Check sheet for the modelled part. Datum: model origin and axes. Units: mm. A direction names the side the tool comes from. Give positions to 0.01 mm unless a question says otherwise; leave off trailing zeros. Loops run counter-clockwise (first coordinate to the right, second up) from the corner with the lowest first, then second, coordinate; pieces in that order, holes last. Notation, with made-up numbers: (13, -13.75) - (60, -13.75) arc R29 cw to (60, 24.25) - close; hole circle Ø7 at (-26, -9). An arc over 180 degrees is marked (long way). Answer in a Markdown table with one row per item. Add a question column.
(1) Sectioned sample at D-D on z = 20.5. Enter the section's corners in (x, y).
(2) Sectioned sample at C-C on y = 13. Enter the section's corners in (x, z), then the cut area to 3 significant figures.
(3) Go/stop test with flat-tipped pins: P1, Ø2, axis at y = 8, z = 2.5, coming from the +X side; P2, Ø2, axis at y = -5.5, z = 3.5, coming from the -X side; P3, Ø1, axis at x = -4, y = -6, coming from the +Z side; P4, Ø1.5, axis at x = -2, y = -3.5, coming from the -Z side. Record where each tip stops, or that it passes through.
(4) Sectioned sample at A-A on z = 6. Enter the section's corners in (x, y), then the cut area to 3 significant figures.
(5) Sectioned sample at B-B on y = -3.25. Enter the section's corners in (x, z), then the cut area to 3 significant figures.
(6) Set-up check for faces 4 (the face through (-6, 1, 11)), 5 (the face through (3.624, -1.945, 0.493)), 6 (the face through (-0.617, -5.4, 0.5)): record each of +Z, -Z, +X, -X, +Y, -Y from which the full face is reachable in a straight line by a thin tool's end or side.
(7) Thickness scan on L1, parallel to Z at x = -6.5, y = 9; L2, parallel to Z at x = -6.25, y = 5; L3, parallel to X at y = 8.75, z = 3.75. Record the ranges inside material, lowest first.
(8) Draft check along Y on faces 1 (the face through (-1, 11, 0)), 2 (the face through (-4.67, 4.6, 0.49)), 3 (the face through (-4.43, 12.34, 10.49)). Enter one of: released by +Y, released by -Y, zero draft, split by the parting line, or undercut.
Autodesk Inventor part; units mm, degrees
ref_plane "YZ Plane" through (0, 0, 0) normal (1, 0, 0) x (0, 1, 0)
ref_plane "XZ Plane" through (0, 0, 0) normal (0, 1, 0) x (-1, 0, 0)
ref_plane "XY Plane" through (0, 0, 0) normal (0, 0, 1) x (1, 0, 0)
sketch "Sketch1" plane through (0, 0, 0) normal (0, 0, 1) x (1, 0, 0)
  line L0 (7.712, 5.2132) -> (7.712, 6.1786)
  line L1 (7.712, 5.2132) -> (-0.617, 1.7442)
  line L2 (7.712, 6.1786) -> (-0.617, 2.7096)
  line L3 (-0.617, 7.1917) -> (7.712, 10.6607)
  line L4 (7.712, 10.6607) -> (-0.5182, 14.502)
  line L5 (-8.8472, 2.0687) -> (-8.8472, 6.5508)
  line L6 (-8.8472, 11.033) -> (-0.617, 7.1917)
  line L7 (-0.5182, 14.502) -> (-8.8472, 11.033)
  line L8 (-0.617, 2.7096) -> (-8.8472, 6.5508)
  line L9 (7.748, -0.2344) -> (7.748, 0.731)
  line L10 (-0.617, 1.7442) -> (-0.617, -1.7726)
  line L11 (7.748, 0.731) -> (-0.5892, -2.738)
  line L12 (7.748, -0.2344) -> (-0.617, -3.7034)
  line L13 (-0.617, -1.7726) -> (-8.8472, 2.0687)
  line L14 (-0.5892, -2.738) -> (-8.8472, 1.1033)
  line L15 (-8.8472, -4.2851) -> (-8.8472, 1.1033)
  line L16 (7.748, -4.7166) -> (7.748, -3.7512)
  line L17 (7.748, -3.7512) -> (-0.617, -7.2201)
  line L18 (-0.617, -8.1855) -> (7.748, -4.7166)
  line L19 (-0.617, -3.7034) -> (-0.617, -7.2201)
  line L20 (-0.617, -8.1855) -> (-8.8472, -4.2851)
  point P0 (0, 0)
extrude "Extrusion1" add sketch "Sketch1" along normal blind 1
sketch "Sketch2" plane through (0, 0, 1) normal (0, 0, 1) x (1, 0, 0)
  line L0 (-0.617, 7.1917) -> (7.712, 10.6607)
  line L1 (7.712, 10.6607) -> (-0.5182, 14.502)
  line L2 (-0.5182, 14.502) -> (-8.8472, 11.033)
  line L3 (-8.8472, 11.033) -> (-0.617, 7.1917)
  line L4 (7.748, -0.2344) -> (7.748, 0.731)
  line L5 (7.748, 0.731) -> (-0.5892, -2.738)
  line L6 (-0.5892, -2.738) -> (-8.8472, 1.1033)
  line L7 (-8.8472, 1.1033) -> (-8.8472, -4.2851)
  line L8 (-8.8472, -4.2851) -> (-0.617, -8.1855)
  line L9 (-0.617, -8.1855) -> (7.748, -4.7166)
  line L10 (7.748, -4.7166) -> (7.748, -3.7512)
  line L11 (7.748, -3.7512) -> (-0.617, -7.2201)
  line L12 (-0.617, -7.2201) -> (-0.617, -3.7034)
  line L13 (-0.617, -3.7034) -> (7.748, -0.2344)
  line L14 (-8.8472, 11.033) -> (-8.8472, 1.1033)
  line L15 (7.712, 10.6607) -> (7.748, -3.7512)
  point P0 (0, 0)
extrude "Extrusion2" add sketch "Sketch2" along normal blind 10 contours L3 L2 L1 L0 | L0 L15 L5 L6 L14 L3 | L15 L13 L12 L11 L10 L9 L8 L7 L6 L5 | L15 L11 L12 L13
sketch "Sketch3" plane through (0, 0, 11) normal (0, 0, 1) x (1, 0, 0)
  circle A0 centre (-0.2029, 3.5969) radius 4.8142
  point P0 (0, 0)
extrude "Extrusion3" add sketch "Sketch3" along normal blind 12
fillet "Fillet1" radius 2 1 edges at (-5.0171, 3.5969, 23)
chamfer "Chamfer1" distance 1 angle 45 7 edges at (-8.8472, 3.374, 11) (-4.7321, -6.2353, 11) (3.5655, -6.451, 11) (7.73, 3.4548, 11) (3.5969, 12.5813, 11) (-4.6827, 12.7675, 11) (-5.0171, 3.5969, 11)
properties part number "stamp"
Reply:
| question | item | result |
|---|---|---|
| 1 | outline | circle Ø9.63 at (-0.2, 3.6) |
| 2 | outline | (-4.12, 0) - (2.7, 0) - (2.7, 10) - (0.34, 11) - (-1.52, 11) - (-4.12, 10) - close |
| 2 | area | 72.6 mm^2 |
| 3 | P1 | x = 7.72 |
| 3 | P2 | x = -8.39 |
| 3 | P3 | z = 11 |
| 3 | P4 | z = 0 |
| 4 | outline | (-8.85, -4.29) - (-0.62, -8.19) - (7.75, -4.72) - (7.75, -3.75) - (7.71, 10.66) - (-0.52, 14.5) - (-8.85, 11.03) - close |
| 4 | area | 315 mm^2 |
| 5 | outline | (-8.85, 0) - (0.48, 0) - (0.48, 1) - (7.75, 1) - (7.75, 10) - (6.75, 11) - (-7.85, 11) - (-8.85, 10) - close |
| 5 | area | 174 mm^2 |
| 6 | face 4 | +Z |
| 6 | face 5 | -Z, +X |
| 6 | face 6 | -Z |
| 7 | L1 | 1 to 11 |
| 7 | L2 | 0 to 11 |
| 7 | L3 | -8.85 to 7.72 |
| 8 | face 1 | zero draft |
| 8 | face 2 | undercut |
| 8 | face 3 | released by +Y |
